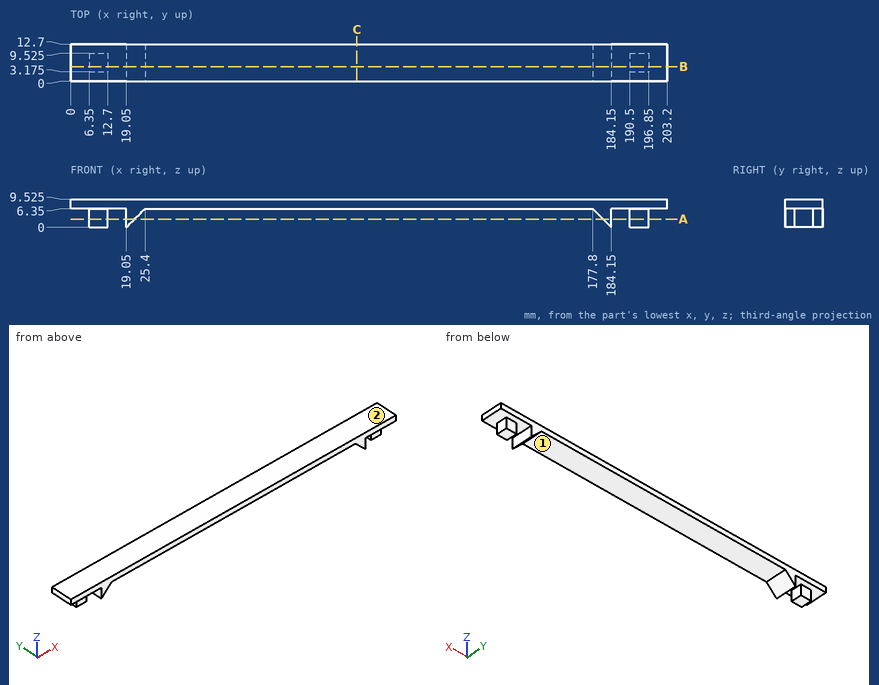
Study the drawing (mm; zero at the part's minimum x, y, z) and answer. Coordinates: 2 decimals unless noted, no trailing zeros. Order: outer loops, then holes, each group sorted by start corner. A loop starts at its lowest first (then second) coordinate and runs counter-clockwise, first axis right, second up. Notation, with made-up numbers: M 46.25,-39 L 71.25,-39 A13 cw 71.25,-28 Z; hole C 50,35 d4. An arc over 180 degrees is marked long. Answer as a JSON object with one key per item and string values. Group by question number.
1. Flat-ended cylindrical pins translate along their axes: P1, Ø3, axis at y = 7.5, z = 2, coming from the -X side; P2, Ø3, axis at x = 193.5, z = 4, coming from the -Y side (3 decimals); P3, Ø1.9, axis at x = 9.5, z = 3, coming from the +Y side (3 decimals). Find the tip coordinate at first contact, or state that the pin passes through.
2. Section C-C on x = 97.5 is taken. Write down the section's boundary in (y, z) (3 decimals), then the cut area to 3 significant figures.
3. Determine the mould class of the marked faces 1 and 2 for opening direction X: released by +X, released by -X, zero draft, split by the parting line, or undercut.
4. Section A-A on z = 2.75 is taken. Write down the section's boundary in (x, y) (3 decimals).
5. Straight lines are drawn through the part: line 1 (X direction, y = 8.75, z = 0.75); line 2 (X direction, y = 4, z = 1.25); line 3 (Z direction, x = 69, y = 9.25) (3 decimals). For each, find the intervals that lie inside material, in ascending order.
6. Section B-B on y = 5 is taken. Write down the section's boundary in (x, z) (3 decimals), then the cut area to 3 significant figures.
Values follow:
{
 "1": {"P1": "x = 6.35", "P2": "y = 3.175", "P3": "y = 9.525"},
 "2": {"outline": "M 0,6.35 L 12.7,6.35 L 12.7,9.525 L 0,9.525 Z", "area": "40.3 mm2"},
 "3": {"face 1": "undercut", "face 2": "zero draft"},
 "4": {"outline": "M 6.35,3.175 L 12.7,3.175 L 12.7,9.525 L 6.35,9.525 Z; M 19.05,0 L 21.8,0 L 21.8,12.7 L 19.05,12.7 Z; M 181.4,0 L 184.15,0 L 184.15,12.7 L 181.4,12.7 Z; M 190.5,3.175 L 196.85,3.175 L 196.85,9.525 L 190.5,9.525 Z"},
 "5": {"line 1": "6.35 to 12.7, 19.05 to 19.8, 183.4 to 184.15, 190.5 to 196.85", "line 2": "6.35 to 12.7, 19.05 to 20.3, 182.9 to 184.15, 190.5 to 196.85", "line 3": "6.35 to 9.525"},
 "6": {"outline": "M 0,6.35 L 6.35,6.35 L 6.35,0 L 12.7,0 L 12.7,6.35 L 19.05,6.35 L 19.05,0 L 25.4,6.35 L 177.8,6.35 L 184.15,0 L 184.15,6.35 L 190.5,6.35 L 190.5,0 L 196.85,0 L 196.85,6.35 L 203.2,6.35 L 203.2,9.525 L 0,9.525 Z", "area": "766 mm2"}
}
